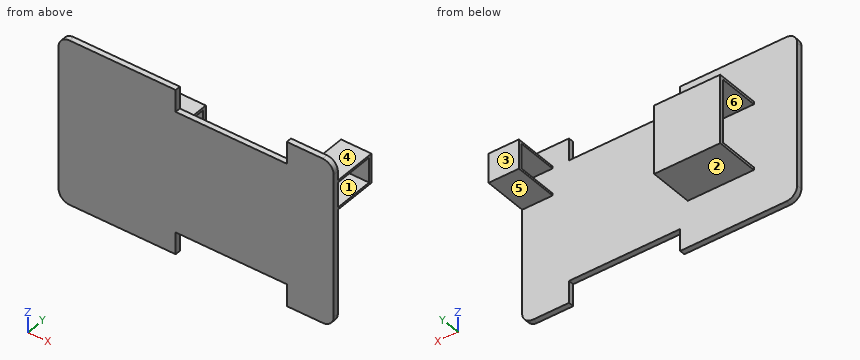
from build123d import *

# Parameters (mm, degrees)
BOSS_EXTRUDE1_DEPTH = 5
SKETCH2_W           = 27.600843984
SKETCH2_H           = 2
SKETCH2_W_2         = 60
SKETCH2_H_2         = 2.5
BOSS_EXTRUDE2_DEPTH = 40
SKETCH4_W           = 27.600843984
SKETCH4_H           = 2.834104075
BOSS_EXTRUDE4_DEPTH = 22.691339628
SKETCH5_W           = 60
SKETCH5_H           = 3.359629359
BOSS_EXTRUDE5_DEPTH = 57.5
FILLET1_R           = 10


with BuildPart() as part:
    # Sketch1 → Boss-Extrude1 (new body)
    with BuildSketch(Plane(origin=(0, 0, 0), x_dir=(1, 0, 0), z_dir=(0, 1, 0))):
        Polygon((106.407471576, 20), (207.407471576, 20), (207.407471576, 0), (250, 0), (250, 150), (207.407471576, 150), (207.407471576, 130), (106.407471576, 130), (106.407471576, 150), (0, 150), (0, 0), (106.407471576, 0), align=None)
    extrude(amount=BOSS_EXTRUDE1_DEPTH)

    # Sketch2 → Boss-Extrude2 (add)
    with BuildSketch(Plane(origin=(0, 5, 0), x_dir=(1, 0, 0), z_dir=(0, 1, 0))):
        with Locations((236.181530472, 44.106973221)):
            Rectangle(SKETCH2_W, SKETCH2_H)
        with Locations((236.181530472, 19.415633593)):
            Rectangle(SKETCH2_W, SKETCH2_H)
        with Locations((69.460984605, 106.25)):
            Rectangle(SKETCH2_W_2, SKETCH2_H_2)
        with Locations((69.460984605, 46.25)):
            Rectangle(SKETCH2_W_2, SKETCH2_H_2)
    extrude(amount=BOSS_EXTRUDE2_DEPTH)

    # Sketch4 → Boss-Extrude4 (add)
    with BuildSketch(Plane.XY.offset(-43.106973221)):
        with Locations((236.181530472, 43.582947963)):
            Rectangle(SKETCH4_W, SKETCH4_H)
    extrude(amount=BOSS_EXTRUDE4_DEPTH)

    # Sketch5 → Boss-Extrude5 (add)
    with BuildSketch(Plane(origin=(0, 0, -47.5), x_dir=(-1, 0, 0), z_dir=(0, 0, -1))):
        with Locations((-69.460984605, 43.320185321)):
            Rectangle(SKETCH5_W, SKETCH5_H)
    extrude(amount=BOSS_EXTRUDE5_DEPTH)

    # Fillet1
    fillet1_edges = [part.edges().sort_by_distance(p)[0] for p in [
        (0, 2.5, -150),
        (250, 2.5, -150),
        (250, 2.5, 0),
        (0, 2.5, 0),
    ]]
    fillet(fillet1_edges, radius=FILLET1_R)


solid = part.part
Build history of the part. All positions in model axes, mm. Face numbers are marked on the shaded views. A direction names the side the tool comes from. Coordinates: 2 decimals unless noted, no trailing zeros. Order: outer loops, then holes, each group sorted by start corner. A loop starts at its lowest first (then second) coordinate and runs counter-clockwise, first axis right, second up. Notation, with made-up numbers: (-9, 42.5) - (33, 42.5) arc R17 cw to (33, 59.5) - close; hole circle Ø8 at (43, -35). An arc over 180 degrees is marked (long way). Put each result on its own line as item: value.
1. Saw through at C-C (x = 94.5). Write the cut outline in (y, z).
Answer sheet:
outline: (0, -150) - (5, -150) - (5, -107.5) - (45, -107.5) - (45, -45) - (5, -45) - (5, 0) - (0, 0) - close; hole (5, -105) - (41.64, -105) - (41.64, -47.5) - (5, -47.5) - close
2. Saw through at D-D (z = -96.5). Write the cut outline in (x, y).
Answer sheet:
outline: (0, 0) - (250, 0) - (250, 5) - (0, 5) - close; (39.46, 41.64) - (99.46, 41.64) - (99.46, 45) - (39.46, 45) - close
3. Saw through at A-A (z = -133.5). Write the cut outline in (x, y), and give its area (3 significant figures).
Answer sheet:
outline: (0, 0) - (106.41, 0) - (106.41, 5) - (0, 5) - close; (207.41, 0) - (250, 0) - (250, 5) - (207.41, 5) - close
area: 745 mm^2
4. Saw through at B-B (y = 26.5). Write the cut outline in (x, z).
Answer sheet:
outline: (39.46, -107.5) - (99.46, -107.5) - (99.46, -105) - (39.46, -105) - close; (39.46, -47.5) - (99.46, -47.5) - (99.46, -45) - (39.46, -45) - close; (222.38, -45.11) - (249.98, -45.11) - (249.98, -43.11) - (222.38, -43.11) - close; (222.38, -20.42) - (249.98, -20.42) - (249.98, -18.42) - (222.38, -18.42) - close
5. Pull direction Z, two halves, no side cores. Call the marked faces 4, 5 and 6: pulls with the +Z half, pulls with the -Z half, needs draft (parallel to the pull), parting line crosses it, or undercut.
Answer sheet:
face 4: pulls with the +Z half
face 5: pulls with the -Z half
face 6: undercut
6. Tool access for the marked faces 1, 2 and 3: list every direction of +Z, -Z, +X, -X, +Y, -Y with a clear straight run to the whole face (end or side of a thin tool).
Answer sheet:
face 1: +X, -X
face 2: -Z, +X, -X, +Y
face 3: +Z, -Z, +X, -X, +Y
7. Probe line 1 along Z through (x, y) = (93.5, 15); line 2 along Y through (x, z) = (48, -56.5); line 3 along Y through (x, z) = (32, -65.5). List the from-to ranges inside material, lowest first. Write a range as [from, to].
Answer sheet:
line 1: z = [-107.5, -105], [-47.5, -45]
line 2: y = [0, 5], [41.64, 45]
line 3: y = [0, 5]
8. Drop flat-ended pins along their axis: P1, Ø1.5, axis at y = 3.5, z = -9, coming from the +X side; P2, Ø1, axis at x = 39, y = 12, coming from the -Z side; P3, Ø22, axis at x = 230, y = 26, coming from the -Z side; P4, Ø5, axis at y = 35, z = -101, coming from the -X side. Give the stop position or say it passes through.
Answer sheet:
P1: stops at x = 250
P2: stops at z = -107.5
P3: stops at z = -45.11
P4: passes through
